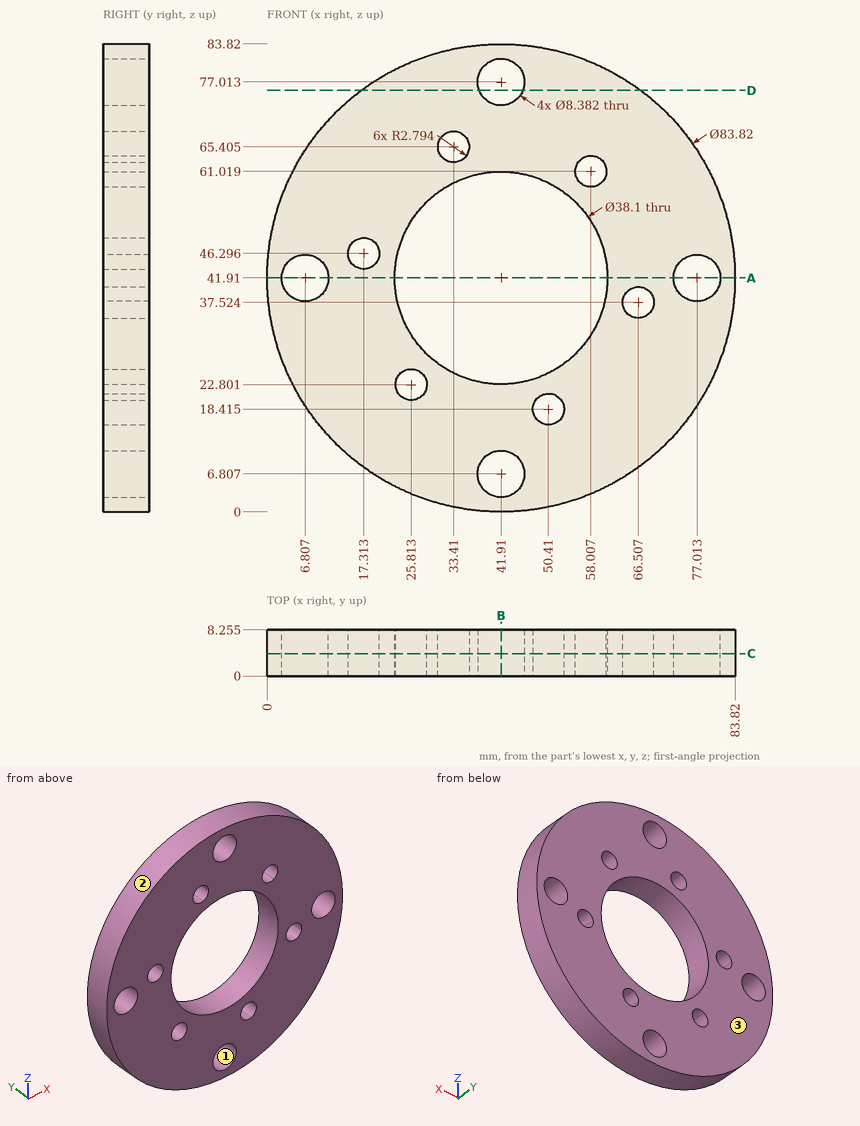
Could you check a few things on this drawing? It's one solid part, dimensions in mm from its lowest x, y, z. Coordinates: 2 decimals unless noted, no trailing zeros. Order: outer loops, then holes, each group sorted by start corner. A loop starts at its lowest first (then second) coordinate and runs counter-clockwise, first axis right, second up. Notation, with made-up numbers: M 81,54.5 L 130,54.5 A14 ccw 130,60.5 Z; hole C 45.25,62.5 d9. An arc over 180 degrees is marked long. Use one line per item in the form item = value. Start each with the question number.
1. Please list where these lines run through material, in increasing order: line 1 (Z direction, x = 41.91, y = 6.5); line 2 (Z direction, x = 48, y = 1) (1 decimal).
2. We'd pull the mould along X, two halves only. Please class the marked faces 1, 2 and 3: +X half, -X half, draft (parallel to the pull), parting line (faces both ways), or undercut.
3. Suppose I cut it at C-C on y = 4. Count the separate pieces of the cut face and the enclosed holes in it, then the cut area to 3 significant figures.
4. Suppose I cut it at B-B on x = 41.91. Write out the boundary of the cut face in (y, z) (1 decimal), then the cut area to 3 significant figures.
5. For pin 1 (1.5 mm diameter, centred on x = 17, y = 4, fed in from +Z) (1 decimal); pin 2 (4 mm diameter, centred on x = 58, y = 3.5, fed in from +Z); pin 3 (4 mm diameter, centred on x = 55, y = 6.5, fed in from +Z); pin 4 (5 mm diameter, centred on x = 41.91, z = 6.81, fed in from -Y) (3 decimals), each with a flat end and sliding along its axis, tell me the tip position at first contact or that it passes through.
6. Suppose I cut it at D-D on z = 75.5. Write out the boundary of the cut face in (x, y) (1 decimal), then the cut area to 3 significant figures.
7. Suppose I cut it at A-A on z = 41.91. Write out the boundary of the cut face in (x, y) (1 decimal), then the cut area to 3 significant figures.
Geometry says:
q1.line_1 = 0 to 2.62, 11 to 22.86, 60.96 to 72.82, 81.2 to 83.82
q1.line_2 = 0.4 to 17, 19.8 to 23.9, 60 to 83.4
q2.face_1 = undercut
q2.face_2 = parting line
q2.face_3 = draft
q3.separate_pieces = 1
q3.enclosed_holes = 11
q3.area = 4,010 mm^2
q4.outline = M 0,0 L 8.3,0 L 8.3,2.6 L 0,2.6 Z; M 0,11 L 8.3,11 L 8.3,22.9 L 0,22.9 Z; M 0,61 L 8.3,61 L 8.3,72.8 L 0,72.8 Z; M 0,81.2 L 8.3,81.2 L 8.3,83.8 L 0,83.8 Z
q4.area = 239 mm^2
q5.pin_1 = 76.2
q5.pin_2 = 81.38
q5.pin_3 = 82.33
q5.pin_4 = through
q6.outline = M 16.8,0 L 38,0 L 38,8.3 L 16.8,8.3 Z; M 45.8,0 L 67,0 L 67,8.3 L 45.8,8.3 Z
q6.area = 349 mm^2
q7.outline = M 0,0 L 2.6,0 L 2.6,8.3 L 0,8.3 Z; M 11,0 L 22.9,0 L 22.9,8.3 L 11,8.3 Z; M 61,0 L 72.8,0 L 72.8,8.3 L 61,8.3 Z; M 81.2,0 L 83.8,0 L 83.8,8.3 L 81.2,8.3 Z
q7.area = 239 mm^2
